Part model, mm, in its own coordinate system. A direction names the side the tool comes from. Round coordinates to 2 decimals unless told otherwise and drop trailing zeros. Loops run counter-clockwise (first coordinate to the right, second up) from the corner with the lowest first, then second, coordinate; pieces in that order, holes last. Notation, with made-up numbers: (27, 70) -> (66, 70) arc R25 cw to (66, 105) -> close; hole circle Ø7 at (87.25, -15.75). An arc over 180 degrees is marked (long way). Use a Markdown table: item, result. Add a question column.
Item 1: Cut at C-C, the plane y = -18.25. List the corners of the cut face in (x, z), plus the area to 3 significant figures.
Item 2: Cut at A-A, the plane z = -8. List the corners of the cut face in (x, y), plus the area to 3 significant figures.
Item 3: Cut at D-D, the plane y = -2. List the corners of the cut face in (x, z), plus the area to 3 significant figures.
Item 4: Flat gauge pin, fed straight in: pin 1 (5 mm diameter, centred on x = 4.5, z = -15.5, fed in from +Y). Where does the tip first touch, or does it go through?
Item 5: Which spindle directions (+Z, -Z, +X, -X, +Y, -Y) get a long thin tool onto all of the face, cutting with end or side? Do faces 1 (the face through (27.171, -13, 0)), 2 (the face through (-2, -13, 18.961)). Say none if no direction does.
Item 6: Cut at B-B, the plane x = 17.5. List the corners of the cut face in (y, z).
Item 7: Probe line 1 (Z direction, x = 10, y = -12.25); line 2 (X direction, y = -8.5, z = 18.5); line 3 (Z direction, x = -25.5, y = -7.75). List the from-to ranges inside material, lowest first. Write a range as [from, to].
```python
from build123d import *

# Parameters (mm, degrees)
F0_W         = 57.346759364
F0_H         = 47.0794383436
F1_DEPTH     = 25.4
F2_R         = 5.08
F3_T1_DEPTH  = 33.02
F3_T3_DEPTH  = 72.4794383436
F3_S7_W      = 5.08
F3_S7_H      = 5.08
F3_T8_DEPTH  = 5.08
F3_S13_W     = 5.08
F3_S13_H     = 5.08
F3_T14_DEPTH = 5.08
F4_T1_DEPTH  = 47.186759364
F4_T3_DEPTH  = 15.24
F4_T5_DEPTH  = 54.6994383436
F4_S9_W      = 5.08
F4_S9_H      = 5.08
F4_T10_DEPTH = 5.08
F4_S15_W     = 5.08
F4_S15_H     = 5.08
F4_T16_DEPTH = 5.08
F4_S21_W     = 5.08
F4_S21_H     = 5.08
F4_T22_DEPTH = 5.08
F5_T1_DEPTH  = 47.186759364
F5_T3_DEPTH  = 15.24
F5_S7_W      = 5.08
F5_S7_H      = 5.08
F5_T8_DEPTH  = 5.08
F5_S13_W     = 5.08
F5_S13_H     = 5.08
F5_T14_DEPTH = 5.08
F5_T18_ANGLE = 89.9999999979
F6_DEPTH     = 25.4


# Not quite as in the source:
# - a fillet or chamfer that OpenCascade refuses, or shapes differently, is made with other operations: its cross-section is extruded or revolved along the edge and cut away or added


with BuildPart() as f1:
    # F0 (on Front) → F1 (new body)
    with BuildSketch(Plane.XZ):
        with Locations((-1.5025353059, 0.5008457229)):
            Rectangle(F0_W, F0_H)
    extrude(amount=F1_DEPTH)

    # F2
    f2_edges = [f1.edges().sort_by_distance(p)[0] for p in [
        (-30.175915, -25.4, 0.500846),
        (-1.502535, -25.4, -23.038873),
        (27.170844, -25.4, 0.500846),
        (-1.502535, -25.4, 24.040565),
    ]]
    fillet(f2_edges, radius=F2_R)

    # F3: fillet of radius 5.08 on 3 edges, made by hand

    # F3_s2 → F3_t1 (cut)
    with BuildSketch(Plane.XZ.offset(-12.7)):
        with BuildLine():
            ThreePointArc((22.0908443761, 24.0405648947), (25.6829468245, 22.5526673431), (27.1708443761, 18.9605648947))
            Line((27.1708443761, 18.9605648947), (27.1708443761, 24.0405648947))
            Line((27.1708443761, 24.0405648947), (22.0908443761, 24.0405648947))
        make_face()
        with BuildLine():
            ThreePointArc((22.0908443761, -23.038873449), (25.6829468245, -21.5509758974), (27.1708443761, -17.958873449))
            Line((27.1708443761, -17.958873449), (27.1708443761, -23.038873449))
            Line((27.1708443761, -23.038873449), (22.0908443761, -23.038873449))
        make_face()
    extrude(amount=F3_T1_DEPTH, mode=Mode.SUBTRACT)

    # F3_s4 → F3_t3 (cut)
    with BuildSketch(Plane.XY.offset(-35.738873449)):
        with BuildLine():
            ThreePointArc((22.0908443761, 0), (25.6829468245, -1.4878975516), (27.1708443761, -5.08))
            Line((27.1708443761, -5.08), (27.1708443761, 0))
            Line((27.1708443761, 0), (22.0908443761, 0))
        make_face()
    extrude(amount=F3_T3_DEPTH, mode=Mode.SUBTRACT)


with BuildPart() as f3_tool6:
    # F3_s7 → F3_t8 (new body)
    with BuildSketch(Plane.XY.offset(-17.958873449)):
        with Locations((24.6308443761, -22.86)):
            Rectangle(F3_S7_W, F3_S7_H)
    extrude(amount=-F3_T8_DEPTH)

    # F3_s9 → F3_t10 (revolve, cut)
    with BuildSketch(Plane(origin=(22.0908443761, -20.32, -17.958873449), x_dir=(-0.7071067812, 0.7071067812, 0), z_dir=(-0.7071067812, -0.7071067812, 0))):
        with BuildLine():
            ThreePointArc((0, -5.08), (5.08, 0), (0, 5.08))
            Line((0, 5.08), (0, -5.08))
        make_face()
    revolve(axis=Axis((22.0908443761, -20.32, -17.958873449), (0, 0, -1)), mode=Mode.SUBTRACT)


with BuildPart() as f1_1:
    add(f1.part)

    # F3_t5: cut F3_tool6
    add(f3_tool6.part, mode=Mode.SUBTRACT)


with BuildPart() as f3_tool12:
    # F3_s13 → F3_t14 (new body)
    with BuildSketch(Plane.XY.offset(18.9605648947)):
        with Locations((24.6308443761, -22.86)):
            Rectangle(F3_S13_W, F3_S13_H)
    extrude(amount=F3_T14_DEPTH)

    # F3_s15 → F3_t16 (revolve, cut)
    with BuildSketch(Plane(origin=(22.0908443761, -20.32, 18.9605648947), x_dir=(-0.7071067812, 0.7071067812, 0), z_dir=(0.7071067812, 0.7071067812, 0))):
        with BuildLine():
            ThreePointArc((0, -5.08), (5.08, 0), (0, 5.08))
            Line((0, 5.08), (0, -5.08))
        make_face()
    revolve(axis=Axis((22.0908443761, -20.32, 18.9605648947), (0, 0, 1)), mode=Mode.SUBTRACT)


with BuildPart() as f1_2:
    add(f1_1.part)

    # F3_t11: cut F3_tool12
    add(f3_tool12.part, mode=Mode.SUBTRACT)

    # F4: fillet of radius 5.08 on 3 edges, made by hand

    # F4_s2 → F4_t1 (cut)
    with BuildSketch(Plane.YZ.offset(-25.0959149879)):
        with BuildLine():
            ThreePointArc((0, -17.958873449), (-1.4878975516, -21.5509758974), (-5.08, -23.038873449))
            Line((-5.08, -23.038873449), (0, -23.038873449))
            Line((0, -23.038873449), (0, -17.958873449))
        make_face()
    extrude(amount=F4_T1_DEPTH, mode=Mode.SUBTRACT)

    # F4_s4 → F4_t3 (cut)
    with BuildSketch(Plane.XZ.offset(5.08)):
        with BuildLine():
            ThreePointArc((-30.1759149879, -17.958873449), (-28.6880174363, -21.5509758974), (-25.0959149879, -23.038873449))
            Line((-25.0959149879, -23.038873449), (-30.1759149879, -23.038873449))
            Line((-30.1759149879, -23.038873449), (-30.1759149879, -17.958873449))
        make_face()
    extrude(amount=F4_T3_DEPTH, mode=Mode.SUBTRACT)

    # F4_s6 → F4_t5 (cut)
    with BuildSketch(Plane.XY.offset(-17.958873449)):
        with BuildLine():
            ThreePointArc((-30.1759149879, -5.08), (-28.6880174363, -1.4878975516), (-25.0959149879, 0))
            Line((-25.0959149879, 0), (-30.1759149879, 0))
            Line((-30.1759149879, 0), (-30.1759149879, -5.08))
        make_face()
    extrude(amount=F4_T5_DEPTH, mode=Mode.SUBTRACT)


with BuildPart() as f4_tool8:
    # F4_s9 → F4_t10 (new body)
    with BuildSketch(Plane.YZ.offset(-25.0959149879)):
        with Locations((-22.86, -20.498873449)):
            Rectangle(F4_S9_W, F4_S9_H)
    extrude(amount=-F4_T10_DEPTH)

    # F4_s11 → F4_t12 (revolve, cut)
    with BuildSketch(Plane(origin=(-25.0959149879, -20.32, -17.958873449), x_dir=(0, 0.7071067812, 0.7071067812), z_dir=(0, -0.7071067812, 0.7071067812))):
        with BuildLine():
            ThreePointArc((0, -5.08), (5.08, 0), (0, 5.08))
            Line((0, 5.08), (0, -5.08))
        make_face()
    revolve(axis=Axis((-25.0959149879, -20.32, -17.958873449), (-1, 0, 0)), mode=Mode.SUBTRACT)


with BuildPart() as f1_3:
    add(f1_2.part)

    # F4_t7: cut F4_tool8
    add(f4_tool8.part, mode=Mode.SUBTRACT)


with BuildPart() as f4_tool14:
    # F4_s15 → F4_t16 (new body)
    with BuildSketch(Plane.XZ.offset(5.08)):
        with Locations((24.6308443761, -20.498873449)):
            Rectangle(F4_S15_W, F4_S15_H)
    extrude(amount=-F4_T16_DEPTH)

    # F4_s17 → F4_t18 (revolve, cut)
    with BuildSketch(Plane(origin=(22.0908443761, -5.08, -17.958873449), x_dir=(-0.7071067812, 0, 0.7071067812), z_dir=(-0.7071067812, 0, -0.7071067812))):
        with BuildLine():
            ThreePointArc((0, -5.08), (5.08, 0), (0, 5.08))
            Line((0, 5.08), (0, -5.08))
        make_face()
    revolve(axis=Axis((22.0908443761, -5.08, -17.958873449), (0, 1, 0)), mode=Mode.SUBTRACT)


with BuildPart() as f1_4:
    add(f1_3.part)

    # F4_t13: cut F4_tool14
    add(f4_tool14.part, mode=Mode.SUBTRACT)


with BuildPart() as f4_tool20:
    # F4_s21 → F4_t22 (new body)
    with BuildSketch(Plane.YZ.offset(-25.0959149879)):
        with Locations((-2.54, -20.498873449)):
            Rectangle(F4_S21_W, F4_S21_H)
    extrude(amount=-F4_T22_DEPTH)

    # F4_s23 → F4_t24 (revolve, cut)
    with BuildSketch(Plane(origin=(-25.0959149879, -5.08, -17.958873449), x_dir=(0, -0.7071067812, 0.7071067812), z_dir=(0, -0.7071067812, -0.7071067812))):
        with BuildLine():
            ThreePointArc((0, -5.08), (5.08, 0), (0, 5.08))
            Line((0, 5.08), (0, -5.08))
        make_face()
    revolve(axis=Axis((-25.0959149879, -5.08, -17.958873449), (-1, 0, 0)), mode=Mode.SUBTRACT)


with BuildPart() as f1_5:
    add(f1_4.part)

    # F4_t19: cut F4_tool20
    add(f4_tool20.part, mode=Mode.SUBTRACT)

    # F5: fillet of radius 5.08 on 2 edges, made by hand

    # F5_s2 → F5_t1 (cut)
    with BuildSketch(Plane.YZ.offset(-25.0959149879)):
        with BuildLine():
            ThreePointArc((-5.08, 24.0405648947), (-1.4878975516, 22.5526673431), (0, 18.9605648947))
            Line((0, 18.9605648947), (0, 24.0405648947))
            Line((0, 24.0405648947), (-5.08, 24.0405648947))
        make_face()
    extrude(amount=F5_T1_DEPTH, mode=Mode.SUBTRACT)

    # F5_s4 → F5_t3 (cut)
    with BuildSketch(Plane.XZ.offset(5.08)):
        with BuildLine():
            ThreePointArc((-30.1759149879, 18.9605648947), (-28.6880174363, 22.5526673431), (-25.0959149879, 24.0405648947))
            Line((-25.0959149879, 24.0405648947), (-30.1759149879, 24.0405648947))
            Line((-30.1759149879, 24.0405648947), (-30.1759149879, 18.9605648947))
        make_face()
    extrude(amount=F5_T3_DEPTH, mode=Mode.SUBTRACT)


with BuildPart() as f5_tool6:
    # F5_s7 → F5_t8 (new body)
    with BuildSketch(Plane.YZ.offset(-25.0959149879)):
        with Locations((-22.86, 21.5005648947)):
            Rectangle(F5_S7_W, F5_S7_H)
    extrude(amount=-F5_T8_DEPTH)

    # F5_s9 → F5_t10 (revolve, cut)
    with BuildSketch(Plane(origin=(-25.0959149879, -20.32, 18.9605648947), x_dir=(0, 0.7071067812, -0.7071067812), z_dir=(0, 0.7071067812, 0.7071067812))):
        with BuildLine():
            ThreePointArc((0, -5.08), (5.08, 0), (0, 5.08))
            Line((0, 5.08), (0, -5.08))
        make_face()
    revolve(axis=Axis((-25.0959149879, -20.32, 18.9605648947), (-1, 0, 0)), mode=Mode.SUBTRACT)


with BuildPart() as f1_6:
    add(f1_5.part)

    # F5_t5: cut F5_tool6
    add(f5_tool6.part, mode=Mode.SUBTRACT)


with BuildPart() as f5_tool12:
    # F5_s13 → F5_t14 (new body)
    with BuildSketch(Plane.XY.offset(18.9605648947)):
        with Locations((24.6308443761, -2.54)):
            Rectangle(F5_S13_W, F5_S13_H)
    extrude(amount=F5_T14_DEPTH)

    # F5_s15 → F5_t16 (revolve, cut)
    with BuildSketch(Plane(origin=(22.0908443761, -5.08, 18.9605648947), x_dir=(-0.7071067812, -0.7071067812, 0), z_dir=(-0.7071067812, 0.7071067812, 0))):
        with BuildLine():
            ThreePointArc((0, -5.08), (5.08, 0), (0, 5.08))
            Line((0, 5.08), (0, -5.08))
        make_face()
    revolve(axis=Axis((22.0908443761, -5.08, 18.9605648947), (0, 0, 1)), mode=Mode.SUBTRACT)


with BuildPart() as f1_7:
    add(f1_6.part)

    # F5_t11: cut F5_tool12
    add(f5_tool12.part, mode=Mode.SUBTRACT)

    # F5_s17 → F5_t18 (revolve, cut)
    with BuildSketch(Plane.XZ.offset(5.0800000001)):
        with BuildLine():
            ThreePointArc((-30.1759149879, 18.9605648947), (-28.6880174363, 22.5526673431), (-25.0959149879, 24.0405648947))
            Line((-25.0959149879, 24.0405648947), (-30.1759149879, 24.0405648947))
            Line((-30.1759149879, 24.0405648947), (-30.1759149879, 18.9605648947))
        make_face()
    revolve(axis=Axis((-25.0959149878, -5.0800000001, 24.0405648947), (0, 0, -1)), revolution_arc=F5_T18_ANGLE, mode=Mode.SUBTRACT)

    # F6 (cut): a face of the model
    f6_faces = [f1_7.faces().sort_by_distance(p)[0] for p in [
        (-1.5025353059, -25.4, 0.5008457229),
    ]]
    extrude(f6_faces, amount=-F6_DEPTH, mode=Mode.SUBTRACT)


solid = f1_7.part
```
A:
| question | item | result |
|---|---|---|
| 1 | outline | (-30.18, -17.96) arc R5.08 ccw to (-25.1, -23.04) -> (22.09, -23.04) arc R5.08 ccw to (27.17, -17.96) -> (27.17, 18.96) arc R5.08 ccw to (22.09, 24.04) -> (-25.1, 24.04) arc R5.08 ccw to (-30.18, 18.96) -> close; hole (-25.1, -17.96) -> (22.09, -17.96) -> (22.09, 18.96) -> (-25.1, 18.96) -> close |
| 1 | area | 936 mm^2 |
| 2 | outline | (-30.18, -20.32) arc R5.08 ccw to (-25.1, -25.4) -> (-25.1, 0) arc R5.08 ccw to (-30.18, -5.08) -> close; (22.09, -25.4) arc R5.08 ccw to (27.17, -20.32) -> (27.17, -5.08) arc R5.08 ccw to (22.09, 0) -> close |
| 2 | area | 236 mm^2 |
| 3 | outline | (-29.14, -17.96) arc R4.04 ccw to (-25.1, -22) -> (22.09, -22) arc R4.04 ccw to (26.13, -17.96) -> (26.13, 18.96) arc R4.04 ccw to (22.09, 23) -> (-25.1, 23) arc R4.04 ccw to (-29.14, 18.96) -> close; hole (-25.1, -17.96) -> (22.09, -17.96) -> (22.09, 18.96) -> (-25.1, 18.96) -> close |
| 3 | area | 731 mm^2 |
| 4 | pin 1 | stops at y = 0 |
| 5 | face 1 | +Z, -Z, +X, +Y, -Y |
| 5 | face 2 | +Y, -Y |
| 6 | outline | (-25.4, -17.96) arc R5.08 ccw to (-20.32, -23.04) -> (-5.08, -23.04) arc R5.08 ccw to (0, -17.96) -> close; (-25.4, 18.96) -> (0, 18.96) arc R5.08 ccw to (-5.08, 24.04) -> (-20.32, 24.04) arc R5.08 ccw to start |
| 7 | line 1 | z = [-23.04, -17.96], [18.96, 24.04] |
| 7 | line 2 | x = [-30.18, -25.1], [22.09, 27.17] |
| 7 | line 3 | z = [-23.02, 24.02] |
